For this review, use the dimensioned drawing (mm, ordinates from the lowest corner) and the shaded views. Give positions to 0.01 mm unless a question says otherwise; leave off trailing zeros. Loops run counter-clockwise (first coordinate to the right, second up) from the corner with the lowest first, then second, coordinate; pieces in that order, holes last. Notation, with made-up numbers: (-6, 88.5) -> (13, 88.5) arc R21 ccw to (13, 127.5) -> close; hole circle Ø11 at (6, -3.5). An arc over 180 degrees is marked (long way). Write each question's results on one line, items separated by ' | '. Start each with the question number.
Q1. Wall thickness on L1, parallel to X at y = 32, z = 12.5; L2, parallel to X at y = 36, z = 48.5; L3, parallel to X at y = 23, z = 29: over which ranges is each line inside the solid? List them lowest first. Write a range as [from, to].
Q2. We need section A-A (z = 25.4). Write out the cut boundary in (x, y), plus the area to 3 significant figures.
Q3. We need section C-C (y = 38.1). Write out the cut boundary in (x, z), plus the area to 3 significant figures.
Q4. Insertion check: pin 1 Ø23 at (x, y) = (241.3, 38.1) entering from -Z. The pin has a flat end and moves straight along its axis. Give the tip position at first contact, or say it passes through.
Q5. We need section B-B (x = 241.3). Write out the cut boundary in (y, z), plus the area to 3 significant figures.
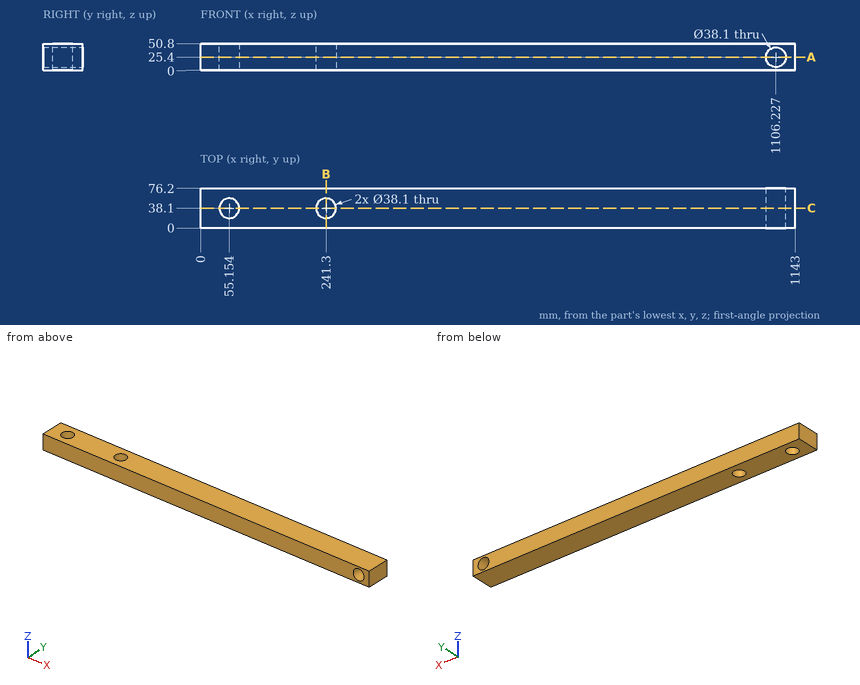
Output:
1) L1: [0, 37.11], [73.2, 223.25], [259.35, 1092.21], [1120.24, 1143] | L2: [0, 36.22], [74.09, 222.37], [260.23, 1143] | L3: [0, 43.54], [66.77, 229.69], [252.91, 1087.52], [1124.93, 1143]
2) outline: (0, 0) -> (1087.18, 0) -> (1087.18, 76.2) -> (0, 76.2) -> close; (1125.28, 0) -> (1143, 0) -> (1143, 76.2) -> (1125.28, 76.2) -> close; hole circle Ø38.1 at (55.15, 38.1); hole circle Ø38.1 at (241.3, 38.1) | area: 81,900 mm2
3) outline: (0, 0) -> (36.1, 0) -> (36.1, 50.8) -> (0, 50.8) -> close; (74.2, 0) -> (222.25, 0) -> (222.25, 50.8) -> (74.2, 50.8) -> close; (260.35, 0) -> (1143, 0) -> (1143, 50.8) -> (260.35, 50.8) -> close; hole circle Ø38.1 at (1106.23, 25.4) | area: 53,100 mm2
4) pin 1: through
5) outline: (0, 0) -> (19.05, 0) -> (19.05, 50.8) -> (0, 50.8) -> close; (57.15, 0) -> (76.2, 0) -> (76.2, 50.8) -> (57.15, 50.8) -> close | area: 1,940 mm2
